Work out the finished part from the listing and answer in its coordinate system (mm). A direction names the side the tool comes from. Coordinates: 2 decimals unless noted, no trailing zeros. Write each loop counter-clockwise with the first axis right and the second up, starting at its lowest first coordinate (ties: lowest second). Pieces come first, ordered by that corner, then holes. Notation, with made-up numbers: M -29,9 L -11,9 A25 ccw -11,29 Z; hole C -25,69.25 d1. An arc over 180 degrees is marked long. Use CSV: the item, a comma, the result in double quotes.
Autodesk Inventor part; units mm, degrees
ref_plane "YZ Plane" through (0, 0, 0) normal (1, 0, 0) x (0, 1, 0)
ref_plane "XZ Plane" through (0, 0, 0) normal (0, 1, 0) x (-1, 0, 0)
ref_plane "XY Plane" through (0, 0, 0) normal (0, 0, 1) x (1, 0, 0)
sketch "Sketch1" plane through (0, 0, 0) normal (0, 0, 1) x (1, 0, 0)
  circle A0 centre (0, 0) radius 7
  dimension "d0" = 14
extrude "Extrusion1" add sketch "Sketch1" along normal blind 25
sketch "Sketch2" plane through (0, 0, 25) normal (0, 0, 1) x (1, 0, 0)
  circle A0 centre (0, 0) radius 2.5
  dimension "d3" = 5
extrude "Extrusion2" cut sketch "Sketch2" against normal up to surface (25 mm away)
sketch "Sketch3" plane through (0, 0, 0) normal (0, 0, -1) x (-1, 0, 0)
  circle A0 centre (0, 0) radius 4
  dimension "d6" = 8
extrude "Extrusion3" cut sketch "Sketch3" against normal blind 12.5
properties part number "Couple"
Item 1: For a pull along X with two mould halves and no side action, classify faces 3 (the face through (6.466, 2.681, 12.325)), 4 (the face through (0, -3, 25)), 5 (the face through (-2, 2, 12.5)) as released by +X, released by -X, zero draft, split by the parting line, or undercut.
Answer:
face 3,"split by the parting line"
face 4,"zero draft"
face 5,"undercut"
Item 2: The part is cut by section A-A (x = 0). Write down the section's boundary in (y, z).
Answer:
outline,"M -7,0 L -4,0 L -4,12.5 L -2.5,12.5 L -2.5,25 L -7,25 Z; M 2.5,12.5 L 4,12.5 L 4,0 L 7,0 L 7,25 L 2.5,25 Z"
Item 3: The part is cut by section D-D (y = -3.5). Write down the section's boundary in (x, z).
Answer:
outline,"M -6.06,0 L -1.94,0 L -1.94,12.5 L 1.94,12.5 L 1.94,0 L 6.06,0 L 6.06,25 L -6.06,25 Z"
Item 4: The part is cut by section C-C (z = 23.5). Write down the section's boundary in (x, y).
Answer:
outline,"C 0,0 d14; hole C 0,0 d5"
Item 5: Consider probe 1 along Y at (x, z) = (0, 9.25); probe 2 along Y at (x, z) = (0, 18.25); probe 3 along X at (y, z) = (-1.5, 23.75). Determine where each line is inside the solid, lowest interval first.
Answer:
probe 1,"y = -7 to -4, 4 to 7"
probe 2,"y = -7 to -2.5, 2.5 to 7"
probe 3,"x = -6.84 to -2, 2 to 6.84"
Item 6: Given pin 1 (6 mm diameter, centred on x = 5.5, z = 14.5, fed in from -Y); pin 2 (1.5 mm diameter, centred on y = 1.5, z = 8, fed in from +X); pin 3 (4 mm diameter, centred on x = -3, z = 6.5, fed in from +Y); pin 4 (3 mm diameter, centred on x = 0, y = 0, fed in from +Z), each flat-ended and moving along its own axis, determine where each tip first touches the part or whether it passes through.
Answer:
pin 1,"stops at y = -6.54"
pin 2,"stops at x = 6.96"
pin 3,"stops at y = 6.93"
pin 4,"passes through"
Item 7: A tool of negligible diameter and unlimited length cuts with its end or side. For faces 1 (the face through (0.867, -3.905, 6.162)), 2 (the face through (-0.54, -2.44, 18.84)), from which of +Z, -Z, +X, -X, +Y, -Y can it reach the whole face along a straight path? Write none if from no direction.
Answer:
face 1,"-Z"
face 2,"+Z, -Z"
